from build123d import *

# Parameters (mm, degrees)
SKETCH1_W           = 7
SKETCH1_H           = 32
BOSS_EXTRUDE1_DEPTH = 2.9
SKETCH2_R           = 0.5
CUT_EXTRUDE1_DEPTH  = 6.8
LPATTERN1_COUNT     = 12
LPATTERN1_PITCH     = 2.54


with BuildPart() as part:
    # Sketch1 → Boss-Extrude1 (new body, symmetric)
    with BuildSketch(Plane(origin=(0, 0, 0), x_dir=(1, 0, 0), z_dir=(0, 1, 0))):
        Rectangle(SKETCH1_W, SKETCH1_H)
    extrude(amount=BOSS_EXTRUDE1_DEPTH, both=True)

    # Sketch2 → Cut-Extrude1 (cut, through all)
    with BuildSketch(Plane(origin=(0, 2.9, 0), x_dir=(1, 0, 0), z_dir=(0, 1, 0))):
        with Locations((0, 13.46)):
            Circle(SKETCH2_R)
    cut_extrude1 = extrude(amount=-CUT_EXTRUDE1_DEPTH, mode=Mode.SUBTRACT)

    # LPattern1: Cut-Extrude1 ×12
    with Locations(*[(0, 0, i * LPATTERN1_PITCH) for i in range(1, LPATTERN1_COUNT)]):
        add(cut_extrude1, mode=Mode.SUBTRACT)


solid = part.part
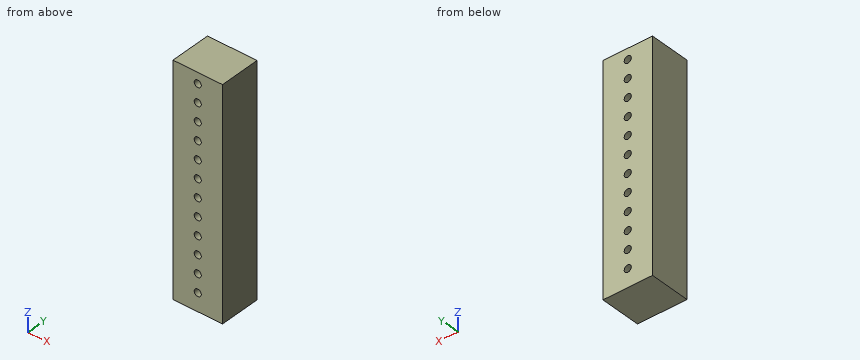
Check sheet for the modelled part. Datum: model origin and axes. Units: mm. Give positions to 0.01 mm unless a question says otherwise; leave off trailing zeros. Loops run counter-clockwise (first coordinate to the right, second up) from the corner with the lowest first, then second, coordinate; pieces in that order, holes last. Notation, with made-up numbers: M 4.25,49 L 40.25,49 A32 cw 40.25,79 Z; hole C 25.25,81 d6. An arc over 180 degrees is marked long. Return JSON: item names as keys, results as strings. Group by question number.
1. Thickness scan on L1, parallel to X at y = 0.5, z = -3.3; L2, parallel to X at y = -2.7, z = 9. Record the ranges inside material, lowest first.
2. Cross-section at A-A on z = 6.86. Record the boundary of the cut face in (x, y).
3. Cross-section at B-B on y = -1.1. State how many separate pieces and enclosed holes the cut face has, plus the area to 3 significant figures.
Return value:
{
 "1": {"L1": "-3.5 to -0.5, 0.5 to 3.5", "L2": "-3.5 to -0.3, 0.3 to 3.5"},
 "2": {"outline": "M -3.5,-2.9 L -0.5,-2.9 L -0.5,2.9 L -3.5,2.9 Z; M 0.5,-2.9 L 3.5,-2.9 L 3.5,2.9 L 0.5,2.9 Z"},
 "3": {"separate pieces": "1", "enclosed holes": "12", "area": "215 mm^2"}
}
